```python
from build123d import *

# Parameters (mm, degrees)
SKETCH1_W            = 82
SKETCH1_H            = 85
BOSS_EXTRUDE1_DEPTH  = 1.2
SKETCH2_W            = 60
SKETCH2_H            = 30
CUT_EXTRUDE1_DEPTH   = 2
SKETCH3_W            = 60
SKETCH3_H            = 15
CUT_EXTRUDE2_DEPTH   = 2
SKETCH4_W            = 82
SKETCH4_H            = 85
SKETCH4_W_2          = 79.6
SKETCH4_H_2          = 82.6
BOSS_EXTRUDE2_DEPTH  = 20
SKETCH5_W            = 62.4
SKETCH5_H            = 17.4
SKETCH5_W_2          = 60
SKETCH5_H_2          = 15
BOSS_EXTRUDE4_DEPTH  = 20
SKETCH10_W           = 1.2
SKETCH10_H           = 3.8
BOSS_EXTRUDE5_DEPTH  = 20
SKETCH11_W           = 5
SKETCH11_H           = 11.2
CUT_EXTRUDE3_DEPTH   = 1.5
SKETCH12_W           = 21.5
SKETCH12_H           = 8
CUT_EXTRUDE4_DEPTH   = 1.5
SKETCH15_W           = 20.5
SKETCH15_H           = 5
CUT_EXTRUDE5_DEPTH   = 1.5
SKETCH16_W           = 79.6
SKETCH16_H           = 1
BOSS_EXTRUDE6_DEPTH  = 1
SKETCH17_W           = 81.6
SKETCH17_H           = 1
BOSS_EXTRUDE7_DEPTH  = 1
SKETCH18_W           = 78.6
SKETCH18_H           = 1
BOSS_EXTRUDE8_DEPTH  = 1
SKETCH19_W           = 80.6
SKETCH19_H           = 1
BOSS_EXTRUDE9_DEPTH  = 1
SKETCH20_W           = 82
SKETCH20_H           = 85
SKETCH20_W_2         = 79.6
SKETCH20_H_2         = 82.6
BOSS_EXTRUDE10_DEPTH = 2.5
SKETCH23_W           = 82.6
SKETCH23_H           = 0.996744569
BOSS_EXTRUDE11_DEPTH = 1
SKETCH25_W           = 78.6
SKETCH25_H           = 0.996744569
BOSS_EXTRUDE13_DEPTH = 1
SKETCH27_W           = 81.6
SKETCH27_H           = 0.996744569
BOSS_EXTRUDE14_DEPTH = 1
CUT_EXTRUDE7_DEPTH   = 1.2


with BuildPart() as part:
    # Sketch1 → Boss-Extrude1 (new body)
    with BuildSketch(Plane(origin=(0, 0, 0), x_dir=(1, 0, 0), z_dir=(0, 1, 0))):
        with Locations((41, 42.5)):
            Rectangle(SKETCH1_W, SKETCH1_H)
    extrude(amount=BOSS_EXTRUDE1_DEPTH)

    # Sketch2 → Cut-Extrude1 (cut)
    with BuildSketch(Plane(origin=(0, 1.2, 0), x_dir=(1, 0, 0), z_dir=(0, 1, 0))):
        with Locations((41, 64.7)):
            Rectangle(SKETCH2_W, SKETCH2_H)
    extrude(amount=-CUT_EXTRUDE1_DEPTH, mode=Mode.SUBTRACT)

    # Sketch3 → Cut-Extrude2 (cut)
    with BuildSketch(Plane(origin=(0, 1.2, 0), x_dir=(1, 0, 0), z_dir=(0, 1, 0))):
        with Locations((41, 37.5)):
            Rectangle(SKETCH3_W, SKETCH3_H)
    extrude(amount=-CUT_EXTRUDE2_DEPTH, mode=Mode.SUBTRACT)

    # Sketch4 → Boss-Extrude2 (add)
    with BuildSketch(Plane.XZ):
        with Locations((41, -42.5)):
            Rectangle(SKETCH4_W, SKETCH4_H)
        with Locations((41, -42.5)):
            Rectangle(SKETCH4_W_2, SKETCH4_H_2, mode=Mode.SUBTRACT)
    extrude(amount=BOSS_EXTRUDE2_DEPTH)

    # Sketch5 → Boss-Extrude4 (add)
    with BuildSketch(Plane.XZ):
        with Locations((41, -37.5)):
            Rectangle(SKETCH5_W, SKETCH5_H)
        with Locations((41, -37.5)):
            Rectangle(SKETCH5_W_2, SKETCH5_H_2, mode=Mode.SUBTRACT)
    extrude(amount=BOSS_EXTRUDE4_DEPTH)

    # Sketch10 → Boss-Extrude5 (add)
    with BuildSketch(Plane.XZ):
        with Locations((9.8, -26.9)):
            Rectangle(SKETCH10_W, SKETCH10_H)
    extrude(amount=BOSS_EXTRUDE5_DEPTH)

    # Sketch11 → Cut-Extrude3 (cut)
    with BuildSketch(Plane.ZY):
        with Locations((-24.5, -9.4)):
            Rectangle(SKETCH11_W, SKETCH11_H)
    extrude(amount=-CUT_EXTRUDE3_DEPTH, mode=Mode.SUBTRACT)

    # Sketch12 → Cut-Extrude4 (cut)
    with BuildSketch(Plane(origin=(0, 0, -85), x_dir=(-1, 0, 0), z_dir=(0, 0, -1))):
        with Locations((-57.4, -4.3)):
            Rectangle(SKETCH12_W, SKETCH12_H)
    extrude(amount=-CUT_EXTRUDE4_DEPTH, mode=Mode.SUBTRACT)

    # Sketch15 → Cut-Extrude5 (cut)
    with BuildSketch(Plane.XY.offset(-45)):
        with Locations((58.25, -2.8)):
            Rectangle(SKETCH15_W, SKETCH15_H)
    extrude(amount=-CUT_EXTRUDE5_DEPTH, mode=Mode.SUBTRACT)

    # Sketch16 → Boss-Extrude6 (add)
    with BuildSketch(Plane.XY.offset(-83.8)):
        with Locations((41, -19.5)):
            Rectangle(SKETCH16_W, SKETCH16_H)
    extrude(amount=BOSS_EXTRUDE6_DEPTH)

    # Sketch17 → Boss-Extrude7 (add)
    with BuildSketch(Plane.ZY.offset(-80.8)):
        with Locations((-42, -19.5)):
            Rectangle(SKETCH17_W, SKETCH17_H)
    extrude(amount=BOSS_EXTRUDE7_DEPTH)

    # Sketch18 → Boss-Extrude8 (add)
    with BuildSketch(Plane(origin=(0, 0, -1.2), x_dir=(-1, 0, 0), z_dir=(0, 0, -1))):
        with Locations((-40.5, -19.5)):
            Rectangle(SKETCH18_W, SKETCH18_H)
    extrude(amount=BOSS_EXTRUDE8_DEPTH)

    # Sketch19 → Boss-Extrude9 (add)
    with BuildSketch(Plane(origin=(1.2, 0, 0), x_dir=(0, 0, -1), z_dir=(1, 0, 0))):
        with Locations((42.5, -19.5)):
            Rectangle(SKETCH19_W, SKETCH19_H)
    extrude(amount=BOSS_EXTRUDE9_DEPTH)

    # Sketch20 → Boss-Extrude10 (add)
    with BuildSketch(Plane.XZ.offset(20)):
        with Locations((41, -42.5)):
            Rectangle(SKETCH20_W, SKETCH20_H)
        with Locations((41, -42.5)):
            Rectangle(SKETCH20_W_2, SKETCH20_H_2, mode=Mode.SUBTRACT)
    extrude(amount=BOSS_EXTRUDE10_DEPTH)

    # Sketch23 → Boss-Extrude11 (add)
    with BuildSketch(Plane.ZY.offset(-80.8)):
        with Locations((-42.5, -22.001627715)):
            Rectangle(SKETCH23_W, SKETCH23_H)
    extrude(amount=BOSS_EXTRUDE11_DEPTH)

    # Sketch25 → Boss-Extrude13 (add)
    with BuildSketch(Plane(origin=(0, 0, -1.2), x_dir=(-1, 0, 0), z_dir=(0, 0, -1))):
        with Locations((-40.5, -22.001627715)):
            Rectangle(SKETCH25_W, SKETCH25_H)
    extrude(amount=BOSS_EXTRUDE13_DEPTH)

    # Sketch27 → Boss-Extrude14 (add)
    with BuildSketch(Plane(origin=(1.2, 0, 0), x_dir=(0, 0, -1), z_dir=(1, 0, 0))):
        with Locations((43, -22.001627715)):
            Rectangle(SKETCH27_W, SKETCH27_H)
    extrude(amount=BOSS_EXTRUDE14_DEPTH)

    # Sketch28 → Cut-Extrude7 (cut)
    with BuildSketch(Plane(origin=(0, 0, -85), x_dir=(-1, 0, 0), z_dir=(0, 0, -1))):
        Polygon((-79.8, -22.5), (-79.8, -21.5), (-80.8, -21.5), (-80.8, -20.2), (-1.2, -20.2), (-1.2, -21.5), (-2.2, -21.5), (-2.2, -22.5), align=None)
    extrude(amount=-CUT_EXTRUDE7_DEPTH, mode=Mode.SUBTRACT)


solid = part.part
```
Verification items for the finished model (mm, model axes). A direction names the side the tool comes from. Give positions to 0.01 mm unless a question says otherwise; leave off trailing zeros. Order: outer loops, then holes, each group sorted by start corner. A loop starts at its lowest first (then second) coordinate and runs counter-clockwise, first axis right, second up. Notation, with made-up numbers: M 44,70.5 L 50,70.5 A19 cw 50,82.5 Z; hole C 54,27 d6. An arc over 180 degrees is marked long. Answer in a Markdown table with one row per item. Add a question column.
Item 1: Scan lines: probe 1 along Z at (x, y) = (50, 0.25); probe 2 along Z at (x, y) = (39.5, -17.5); probe 3 along X at (y, z) = (-7.5, -33). Record each from-to range of solid material in increasing order. Write a range as from..to.
Item 2: Section check C-C, the plane y = -2. Enter the section's corners in (x, z).
Item 3: Section check B-B, the plane z = -66. Enter the section's corners in (x, y), and give its area (3 significant figures).
Item 4: Mould release check, pull along Y, two halves, no side actions. Record for faces 1 (the flat face through (41, -10, -46.2)), 2 (the flat face through (31, -20, -29)), 3 (the flat face through (40, -9, -83.8)): released by +Y, released by -Y, zero draft, split by the parting line, or undercut.
Item 5: Section check D-D, the plane x = 43. State how many separate pieces and enclosed holes the cut face has, and give its area (3 significant figures).
Item 6: Gauge pin test, flat end, axial feed: pin 1 (3 mm diameter, centred on x = 55, y = -8, fed in from -Z). Record the tip position at first contact, or that the pin passes through.
Item 7: Section check A-A, the plane y = -17. Enter the section's corners in (x, z).
Item 8: Tool access check on faces 4 (the flat face through (1.2, -9, -43)), 5 (the flat face through (41, -10, -28.8)), 6 (the flat face through (11, -9, -38)). Record the directions out of +Z, -Z, +X, -X, +Y, -Y that give a thin tool (end or side, any length) a straight path to the whole face; none if there is none.
Filled sheet:
| question | item | result |
|---|---|---|
| 1 | probe 1 | z = -85..-79.7, -49.7..-45, -30..0 |
| 1 | probe 2 | z = -85..-83.8, -46.2..-45, -30..-28.8, -1.2..0 |
| 1 | probe 3 | x = 0..1.2, 9.8..11, 71..72.2, 80.8..82 |
| 2 | outline | M 0,-85 L 46.65,-85 L 46.65,-83.8 L 1.2,-83.8 L 1.2,-1.2 L 80.8,-1.2 L 80.8,-83.8 L 68.15,-83.8 L 68.15,-85 L 82,-85 L 82,0 L 0,0 Z; M 9.2,-28.8 L 9.8,-28.8 L 9.8,-46.2 L 48,-46.2 L 48,-45 L 11,-45 L 11,-30 L 71,-30 L 71,-45 L 68.5,-45 L 68.5,-46.2 L 72.2,-46.2 L 72.2,-28.8 L 10.4,-28.8 L 10.4,-25 L 9.2,-25 Z |
| 3 | outline | M 0,-22.5 L 2.2,-22.5 L 2.2,-21.5 L 1.2,-21.5 L 1.2,-20 L 2.2,-20 L 2.2,-19 L 1.2,-19 L 1.2,0 L 11,0 L 11,1.2 L 0,1.2 Z; M 71,0 L 80.8,0 L 80.8,-19 L 79.8,-19 L 79.8,-20 L 80.8,-20 L 80.8,-21.5 L 79.8,-21.5 L 79.8,-22.5 L 82,-22.5 L 82,1.2 L 71,1.2 Z |
| 3 | area | 84.4 mm^2 |
| 4 | face 1 | zero draft |
| 4 | face 2 | released by -Y |
| 4 | face 3 | undercut |
| 5 | separate pieces | 3 |
| 5 | enclosed holes | 0 |
| 5 | area | 150 mm^2 |
| 6 | pin 1 | stops at z = -85 |
| 7 | outline | M 0,-85 L 82,-85 L 82,0 L 0,0 Z; M 9.2,-28.8 L 9.8,-28.8 L 9.8,-46.2 L 72.2,-46.2 L 72.2,-28.8 L 10.4,-28.8 L 10.4,-25 L 9.2,-25 Z; hole M 1.2,-83.8 L 80.8,-83.8 L 80.8,-1.2 L 1.2,-1.2 Z; hole M 11,-45 L 71,-45 L 71,-30 L 11,-30 Z |
| 8 | face 4 | none |
| 8 | face 5 | -Y |
| 8 | face 6 | +Y, -Y |
